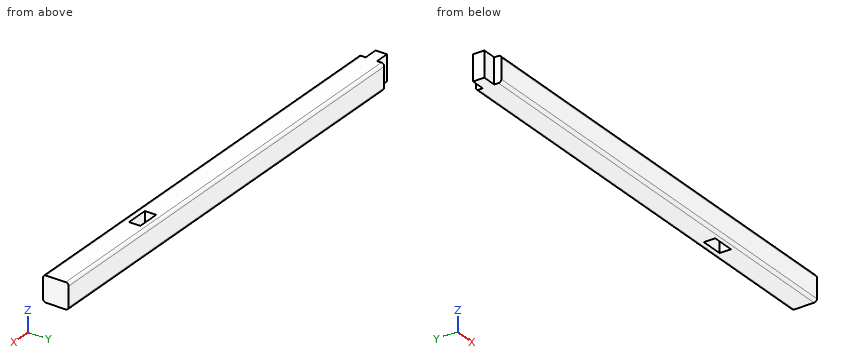
from build123d import *

# Parameters (mm, degrees)
F0_W     = 45
F0_H     = 45
F1_DEPTH = 400
F2_W     = 20
F2_H     = 45
F3_DEPTH = 25
F4_R     = 5
F5_W     = 40
F5_H     = 20
F6_DEPTH = 45.001


with BuildPart() as f1:
    # F0 (on Right) → F1 (new body, symmetric)
    with BuildSketch(Plane.YZ):
        Rectangle(F0_W, F0_H)
    extrude(amount=F1_DEPTH, both=True)

    # F2 (on face) → F3 (join)
    with BuildSketch(Plane(origin=(-400, 0, 0), x_dir=(0, -1, 0), z_dir=(-1, 0, 0))):
        Rectangle(F2_W, F2_H)
    extrude(amount=F3_DEPTH)

    # F4
    f4_edges = [f1.edges().sort_by_distance(p)[0] for p in [
        (0, -22.5, -22.5),
        (0, 22.5, -22.5),
        (0, -22.5, 22.5),
        (0, 22.5, 22.5),
    ]]
    fillet(f4_edges, radius=F4_R)

    # F5 (on face) → F6 (cut, through all)
    with BuildSketch(Plane.XY.offset(22.5)):
        with Locations((180, 0)):
            Rectangle(F5_W, F5_H)
    extrude(amount=-F6_DEPTH, mode=Mode.SUBTRACT)


solid = f1.part
CAD build for the part. Positions are in the model's coordinates, mm. Coordinates: 2 decimals unless noted, no trailing zeros. Loops run counter-clockwise (first coordinate to the right, second up) from the corner with the lowest first, then second, coordinate; pieces in that order, holes last. Notation, with made-up numbers: (10.25, 0) - (60.25, 0) arc R23 cw to (60.25, 28) - close; hole circle Ø1 at (-23, -24). An arc over 180 degrees is marked (long way). Use one line per item in the form item = value. Start each with the question number.
1) Flat gauge pins, fed straight in: pin 1 (8 mm diameter, centred on y = 15, z = 4, fed in from -X); pin 2 (12.5 mm diameter, centred on x = -414.5, z = 10.5, fed in from +Y). Where does each tip first touch, or does it go through?
2) Band-saw the part on B-B (z = 10). Give the cut face in (x, y).
3) Band-saw the part on A-A (y = 3). Give the cut face in (x, z).
4) Drill centre lines: L1, parallel to X at y = 3, z = 11.5; L2, parallel to X at y = 16, z = 10.5; L3, parallel to Y at x = 183, z = 1.5. Where is each one in solid material? Low to high. Write a range as from..to.
Check values:
q1.pin_1 = -400
q1.pin_2 = 10
q2.outline = (-425, -10) - (-400, -10) - (-400, -22.5) - (400, -22.5) - (400, 22.5) - (-400, 22.5) - (-400, 10) - (-425, 10) - close; hole (160, -10) - (200, -10) - (200, 10) - (160, 10) - close
q3.outline = (-425, -22.5) - (160, -22.5) - (160, 22.5) - (-425, 22.5) - close; (200, -22.5) - (400, -22.5) - (400, 22.5) - (200, 22.5) - close
q4.L1 = -425..160, 200..400
q4.L2 = -400..400
q4.L3 = -22.5..-10, 10..22.5
